Answer from the drawing. Dimensions are ordinates in mm from the lowest x, y and z of the part. Round coordinates to 2 decimals unless told otherwise and drop trailing zeros. Order: outer loops, then holes, each group sorted by start corner. A loop starts at its lowest first (then second) coordinate and runs counter-clockwise, first axis right, second up. Notation, with made-up numbers: (-36, -12) -> (-24, -12) arc R12 ccw to (-24, 4) -> close; hole circle Ø11 at (-16.75, -4.5). An arc over 180 degrees is marked (long way). Use a Markdown table: item, result. Add a question column.
1. Section A-A, the plane x = 1.25 is taken. Give the vertices of the cut face in (y, z) (1 decimal).
2. Consider L1, parallel to Y at x = 15.5, z = 0.25 (1 decimal); L2, parallel to Y at x = 13.25, z = 0.15 (1 decimal). Determine where each line is inside the solid, lowest interval first. Write a range as [from, to].
3. Given pin 1 (1.5 mm diameter, centred on x = 6, y = 6.5, fed in from -Z), flat-ended and moving along its own axis, determine where the tip first touches the part or whether it passes through.
4. Section C-C, the plane y = 10.75 is taken. Give the vertices of the cut face in (x, z).
5. Section B-B, the plane z = 0.25 is taken. Give the vertices of the cut face in (x, y) (1 decimal).
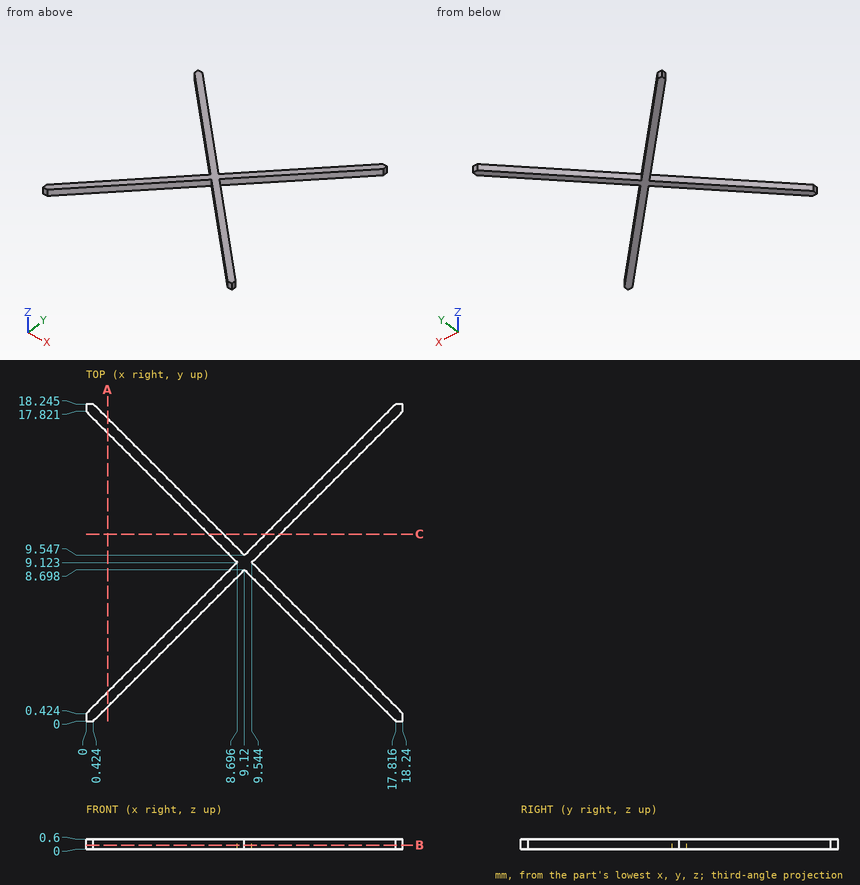
Verdict:
| question | item | result |
|---|---|---|
| 1 | outline | (0.8, 0) -> (1.7, 0) -> (1.7, 0.6) -> (0.8, 0.6) -> close; (16.6, 0) -> (17.4, 0) -> (17.4, 0.6) -> (16.6, 0.6) -> close |
| 2 | L1 | y = [2.3, 3.2], [15.1, 15.9] |
| 2 | L2 | y = [4.6, 5.4], [12.8, 13.7] |
| 3 | pin 1 | stops at z = 0 |
| 4 | outline | (7.07, 0) -> (7.92, 0) -> (7.92, 0.6) -> (7.07, 0.6) -> close; (10.32, 0) -> (11.17, 0) -> (11.17, 0.6) -> (10.32, 0.6) -> close |
| 5 | outline | (0, 0) -> (0.4, 0) -> (9.1, 8.7) -> (17.8, 0) -> (18.2, 0) -> (18.2, 0.4) -> (9.5, 9.1) -> (18.2, 17.8) -> (18.2, 18.2) -> (17.8, 18.2) -> (9.1, 9.5) -> (0.4, 18.2) -> (0, 18.2) -> (0, 17.8) -> (8.7, 9.1) -> (0, 0.4) -> close |
